from build123d import *

# Parameters (mm, degrees)
F0_W        = 20.32
F0_H        = 20.32
F1_DEPTH    = 7.62
F3_DEPTH    = 20.32
F5_D        = 12.7
F5_DEPTH    = 7.62
F5_TIP      = 3.8154649308
F6_T1_DEPTH = 45.72
F6_T3_DEPTH = 45.4214045093
F6_T5_DEPTH = 45.72
F6_T7_DEPTH = 45.7221937612


# Not quite as in the source:
# - a fillet or chamfer that OpenCascade refuses, or shapes differently, is made with other operations: its cross-section is extruded or revolved along the edge and cut away or added


with BuildPart() as f1:
    # F0 (on Front) → F1 (new body)
    with BuildSketch(Plane.XZ):
        with Locations((-2.1305914207, -0.150394626)):
            Rectangle(F0_W, F0_H)
    extrude(amount=F1_DEPTH)

    # F2 (on face) → F3 (join)
    with BuildSketch(Plane.XZ.offset(7.62)):
        Polygon((-12.2905914207, 10.009605374), (-12.2905914207, -10.310394626), (8.0294085793, -10.0117991352), (8.0294085793, 10.009605374), align=None)
    extrude(amount=F3_DEPTH)

    # F5
    with Locations(Plane.XZ.offset(27.94)):
        with Locations((-2.1422964055, 0)):
            Hole(F5_D / 2, depth=F5_DEPTH)
            with Locations((0, 0, -(F5_DEPTH + F5_TIP / 2))):  # 118° drill point
                Cone(0, F5_D / 2, F5_TIP, mode=Mode.SUBTRACT)

    # F6: fillet of radius 5.08 on 4 edges, made by hand

    # F6_s2 → F6_t1 (cut)
    with BuildSketch(Plane.YZ.offset(-24.9905914207)):
        with BuildLine():
            ThreePointArc((-22.86, 10.009605374), (-26.4521024484, 8.5217078225), (-27.94, 4.929605374))
            Line((-27.94, 4.929605374), (-27.94, 10.009605374))
            Line((-27.94, 10.009605374), (-22.86, 10.009605374))
        make_face()
    extrude(amount=F6_T1_DEPTH, mode=Mode.SUBTRACT)

    # F6_s4 → F6_t3 (cut)
    with BuildSketch(Plane.XY.offset(-22.7117991352)):
        with BuildLine():
            ThreePointArc((8.0294085793, -22.86), (6.5415110277, -26.4521024484), (2.9494085793, -27.94))
            Line((2.9494085793, -27.94), (8.0294085793, -27.94))
            Line((8.0294085793, -27.94), (8.0294085793, -22.86))
        make_face()
    extrude(amount=F6_T3_DEPTH, mode=Mode.SUBTRACT)

    # F6_s6 → F6_t5 (cut)
    with BuildSketch(Plane.XY.offset(-23.010394626)):
        with BuildLine():
            ThreePointArc((-7.2105914207, -27.94), (-10.8026938691, -26.4521024484), (-12.2905914207, -22.86))
            Line((-12.2905914207, -22.86), (-12.2905914207, -27.94))
            Line((-12.2905914207, -27.94), (-7.2105914207, -27.94))
        make_face()
    extrude(amount=F6_T5_DEPTH, mode=Mode.SUBTRACT)

    # F6_s8 → F6_t7 (cut)
    with BuildSketch(Plane(origin=(-25.138042131, 0, -0.3693949816), x_dir=(0, 1, 0), z_dir=(0.999892051, 0, 0.0146930737))):
        with BuildLine():
            ThreePointArc((-27.94, -5.0486950632), (-26.4521024484, -8.6407975117), (-22.86, -10.1286950632))
            Line((-22.86, -10.1286950632), (-27.94, -10.1286950632))
            Line((-27.94, -10.1286950632), (-27.94, -5.0486950632))
        make_face()
    extrude(amount=F6_T7_DEPTH, mode=Mode.SUBTRACT)


solid = f1.part
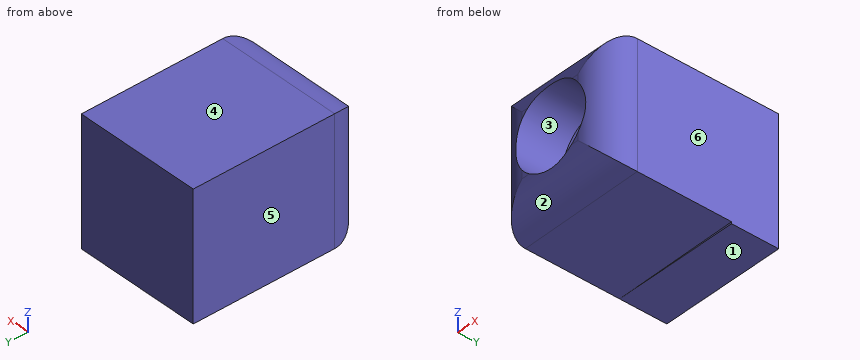
Model file for the job. Use its own axes, mm. Face numbers are marked on the shaded views. A direction names the side the tool comes from. Coordinates: 2 decimals unless noted, no trailing zeros. Write each question's results on one line, items separated by ' | '. Start each with the question number.
1) Mould opens along X. For the marked faces 3, 4, 5 and 6 say: pulls with the +X half, pulls with the -X half, needs draft (parallel to the pull), parting line crosses it, or undercut.
2) 3-axis set-ups, long thin cutter, end or side, ignore diameter. For the marked faces 1 and 2: which of +Z, -Z, +X, -X, +Y, -Y reach the whole face in a straight line?
3) Probe line 1 along X through (y, z) = (-22.5, 0); line 2 along Y through (x, z) = (-7.25, 5); line 3 along X through (y, z) = (-25.25, 0). List the from-to ranges inside material, lowest first. Write a range as from..to.
4) Flat gauge pins, fed straight in: P1, Ø6, axis at x = -7, y = -11.5, coming from the -Z side; P2, Ø12, axis at x = 4, y = -16.5, coming from the -Z side. Where does each tip first touch, or does it go through?
Returned:
1) face 3: undercut | face 4: needs draft | face 5: pulls with the -X half | face 6: pulls with the +X half
2) face 1: -Z, +X, -X, +Y, -Y | face 2: -Z, +X, -Y
3) line 1: -12.29..-8.49, 4.21..8.03 | line 2: -27.94..0 | line 3: -11.69..-8.49, 4.21..7.43
4) P1: z = -10.28 | P2: z = -10.16
